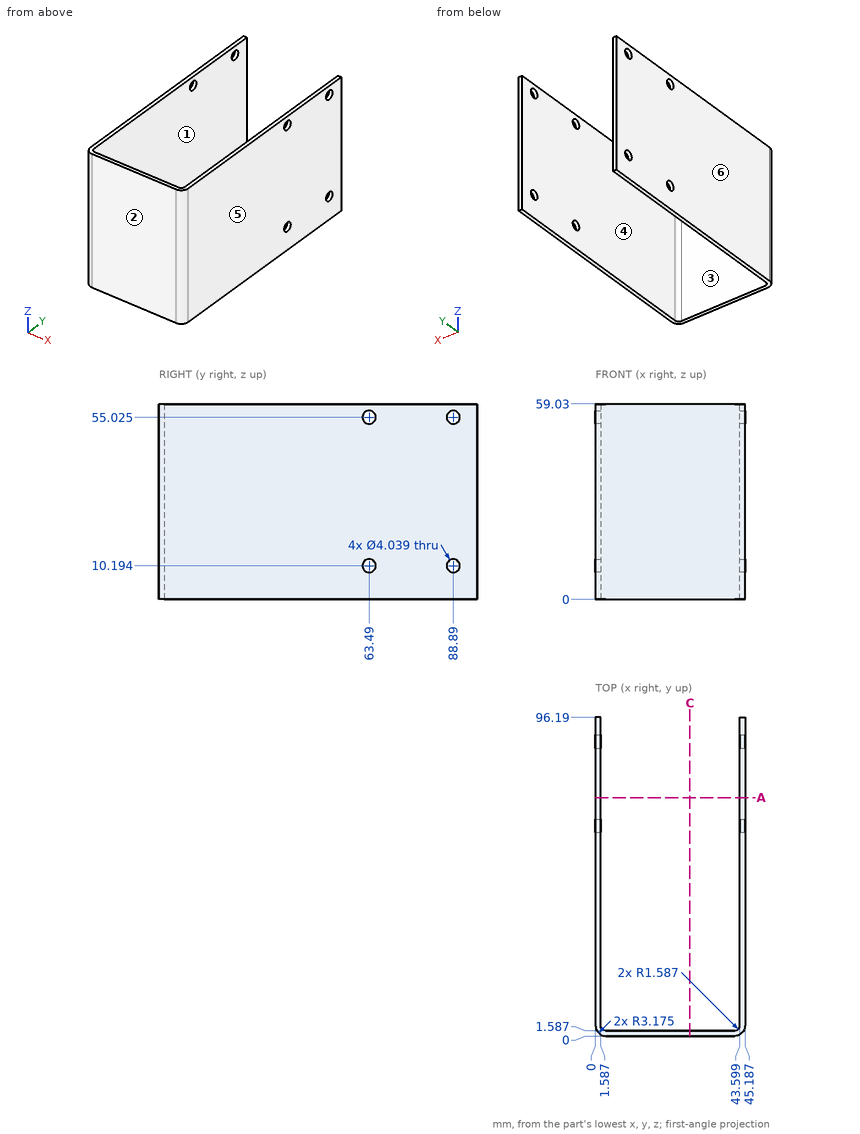
Can you work these out from the drawing? Everything is in mm from the part's minimum corner. A direction names the side the tool comes from. Round coordinates to 2 decimals unless told otherwise and drop trailing zeros. Loops run counter-clockwise (first coordinate to the right, second up) from the corner with the lowest first, then second, coordinate; pieces in that order, holes last. Notation, with made-up numbers: M -24,87.25 L 29,87.25 A22 ccw 29,107.25 Z; hole C -22,62 d4. An arc over 180 degrees is marked long. Answer in a Markdown table with one row per item.
1. I'm going to push flat-ended pins straight in: pin 1 Ø5 at (x, z) = (12, 50.5) entering from +Y; pin 2 Ø3.5 at (y, z) = (88.89, 10.19) entering from -X. Where does each tip first touch, or does it pass through?
Established:
| item | result |
|---|---|
| pin 1 | y = 1.59 |
| pin 2 | through |
2. Thinking about a two-plate mould opening in X: for the marked faces 3, 4, 5 and 6, which applies, pulls with the +X half, pulls with the -X half, needs draft (parallel to the pull), parting line crosses it, or undercut?
Established:
| item | result |
|---|---|
| face 3 | undercut |
| face 4 | undercut |
| face 5 | pulls with the +X half |
| face 6 | pulls with the -X half |
3. On a 3-axis mill with a long thin cutter (end or side, diameter ignored), from which of +Z, -Z, +X, -X, +Y, -Y can I reach the whole of each face in a straight line? I mean the marked faces 1 and 2. Say none if no direction works.
Established:
| item | result |
|---|---|
| face 1 | +Z, -Z, +Y |
| face 2 | +Z, -Z, +X, -X, -Y |
4. Please list where these lines run through material, in increasing order: line 1 (X direction, y = 24, z = 20); line 2 (Y direction, x = 7, z = 5); line 3 (Y direction, x = 43, z = 54.5) (1 decimal). Write a range as from..to.
Established:
| item | result |
|---|---|
| line 1 | 0..1.59, 43.6..45.19 |
| line 2 | 0..1.59 |
| line 3 | 0.2..1.9 |
5. If we section it at A-A, the plane y = 72: Please give me the cut outline in (x, z).
Established:
| item | result |
|---|---|
| outline | M 0,0 L 1.59,0 L 1.59,59.03 L 0,59.03 Z; M 43.6,0 L 45.19,0 L 45.19,59.03 L 43.6,59.03 Z |
6. If we section it at C-C, the plane x = 28.5: Please give me the cut outline in (y, z).
Established:
| item | result |
|---|---|
| outline | M 0,0 L 1.59,0 L 1.59,59.03 L 0,59.03 Z |
